Autodesk Inventor part; units mm, degrees
ref_plane "YZ Plane" through (0, 0, 0) normal (1, 0, 0) x (0, 1, 0)
ref_plane "XZ Plane" through (0, 0, 0) normal (0, 1, 0) x (-1, 0, 0)
ref_plane "XY Plane" through (0, 0, 0) normal (0, 0, 1) x (1, 0, 0)
sketch "스케치1" plane through (0, 0, 0) normal (0, 0, 1) x (1, 0, 0)
  line L0 (0, 0) -> (0, 150)
  line L1 (45, 0) -> (-45, 0)
  line L2 (-45, 0) -> (-45, 10)
  line L3 (-45, 10) -> (45, 10)
  line L4 (45, 10) -> (45, 0)
  line L5 (45, 0) -> (-45, 10) construction
  line L6 (-45, 0) -> (45, 10) construction
  line L7 (-35, 130) -> (35, 130)
  line L8 (35, 130) -> (35, 140)
  line L9 (35, 140) -> (-35, 140)
  line L10 (-35, 140) -> (-35, 130)
  line L11 (-35, 130) -> (35, 140) construction
  line L12 (35, 130) -> (-35, 140) construction
  line L13 (-40, 65) -> (40, 65)
  line L14 (40, 65) -> (40, 75)
  line L15 (40, 75) -> (-40, 75)
  line L16 (-40, 75) -> (-40, 65)
  line L17 (-40, 65) -> (40, 75) construction
  line L18 (40, 65) -> (-40, 75) construction
  line L19 (5, 150) -> (-5, 150)
  line L20 (-5, 0) -> (5, 0)
  line L21 (-45, 10) -> (-40, 10)
  line L22 (-40, 10) -> (-40, 75)
  line L23 (-40, 75) -> (-45, 75)
  line L24 (-45, 75) -> (-45, 10)
  line L25 (45, 10) -> (40, 10)
  line L26 (40, 10) -> (40, 75)
  line L27 (40, 75) -> (45, 75)
  line L28 (45, 75) -> (45, 10)
  line L29 (5, 0) -> (5, 10)
  line L30 (5, 65) -> (5, 150)
  line L31 (-5, 150) -> (-5, 65)
  line L32 (-5, 10) -> (-5, 0)
  line L33 (0, 10) -> (10, 10)
  line L34 (10, 10) -> (10, 65)
  line L35 (10, 65) -> (0, 65)
  line L36 (0, 65) -> (0, 10)
  line L37 (0, 10) -> (-10, 10)
  line L38 (-10, 10) -> (-10, 65)
  line L39 (-10, 65) -> (0, 65)
  line L40 (0, 65) -> (0, 10)
  line L41 (-10, 65) -> (-20, 65)
  line L42 (-20, 65) -> (-20, 10)
  line L43 (-20, 10) -> (-10, 10)
  line L44 (-10, 10) -> (-10, 65)
  line L45 (10, 65) -> (20, 65)
  line L46 (20, 65) -> (20, 10)
  line L47 (20, 10) -> (10, 10)
  line L48 (10, 10) -> (10, 65)
  point P0 (0, 5)
  point P1 (0, 135)
  point P2 (0, 70)
  point P3 (-5, 140)
  point P4 (5, 140)
  point P5 (-5, 75)
  point P6 (5, 75)
  point P7 (-5, 130)
  point P8 (5, 130)
  dimension "d16" = 150
  dimension "d17" = 90
  dimension "d18" = 10
  dimension "d22" = 70
  dimension "d23" = 10
  dimension "d25" = 80
  dimension "d26" = 10
  dimension "d27" = 55
  dimension "d28" = 55
  dimension "d29" = 10
  dimension "d30" = 150
  dimension "d35" = 10
  dimension "d36" = 10
  dimension "d37" = 10
  dimension "d38" = 10
extrude "돌출1" add sketch "스케치1" along normal blind 30 and the other way blind 30 contours L1 L32 L3 L0 | L0 L3 L29 L1 | L29 L3 L4 L1 | L1 L2 L3 L32 | L13 L31 L15 L0 | L0 L15 L30 L13 | L15 L31 L7 L0 | L0 L7 L30 L15 | L13 L16 L15 L31 | L30 L15 L14 L13 | L7 L31 L9 L0 | L0 L9 L30 L7 | L9 L31 L19 L0 | L0 L19 L30 L9 | L7 L10 L9 L31 | L30 L9 L8 L7
extrude "돌출2" add sketch "스케치1" along normal blind 30 and the other way blind 30 contours L3 L26 L14 L27 L28 | L24 L23 L16 L22 L3
extrude "돌출3" add sketch "스케치1" along normal blind 10 and the other way blind 10 contours L3 L42 L13 L38 | L34 L13 L46 L3
properties part number "팔"
Check sheet for the modelled part. Datum: model origin and axes. Units: mm. A direction names the side the tool comes from. Give positions to 0.01 mm unless a question says otherwise; leave off trailing zeros. Write each loop counter-clockwise with the first axis right and the second up, starting at its lowest first coordinate (ties: lowest second). Pieces come first, ordered by that corner, then holes.
Item 1: Scan lines: L1, parallel to Y at x = -24.5, z = -18; L2, parallel to X at y = 10.5, z = -4; L3, parallel to X at y = 30, z = -26.5. Record each from-to range of solid material in increasing order.
Item 2: Cross-section at B-B (z = -13). Enter the section's corners in (x, y), and give its area (3 significant figures).
Item 3: Cross-section at A-A (x = -23). Enter the section's corners in (y, z), and give its area (3 significant figures).
Item 4: Cross-section at D-D (x = -13.5). Enter the section's corners in (y, z).
Item 5: Access from +Z, -Z, +X, -X, +Y, -Y to the whole of each face (thin tool, end or side, straight path). Record for faces 4 (the face through (-20, 130, 0)), 5 (the face through (20, 140, 0)), 6 (the face through (15, 38, 10)).
Item 6: Draft check along Y on faces 1 (the face through (-20, 38, 0)), 2 (the face through (45, 38, 0)), 3 (the face through (-20, 140, 0)). Enter one of: released by +Y, released by -Y, zero draft, split by the parting line, or undercut.
Item 7: Gauge pin test, flat ends, axial feed: pin 1 (15 mm diameter, centred on x = 26, z = -7, fed in from +Y); pin 2 (1 mm diameter, centred on x = 19.5, y = 25, fed in from -Z); pin 3 (5 mm diameter, centred on y = 133.5, z = -0.5, fed in from +X). Record the tip position at first contact, or that the pin passes through.
Item 8: Cross-section at C-C (y = 20). Enter the section's corners in (x, z).
Report:
1. L1: y = 0 to 10, 65 to 75, 130 to 140
1. L2: x = -45 to -40, -20 to -10, 10 to 20, 40 to 45
1. L3: x = -45 to -40, 40 to 45
2. outline: (-45, 0) - (45, 0) - (45, 75) - (5, 75) - (5, 130) - (35, 130) - (35, 140) - (5, 140) - (5, 150) - (-5, 150) - (-5, 140) - (-35, 140) - (-35, 130) - (-5, 130) - (-5, 75) - (-45, 75) - close; hole (-40, 10) - (40, 10) - (40, 65) - (-40, 65) - close
2. area: 3,700 mm2
3. outline: (0, -30) - (10, -30) - (10, 30) - (0, 30) - close; (65, -30) - (75, -30) - (75, 30) - (65, 30) - close; (130, -30) - (140, -30) - (140, 30) - (130, 30) - close
3. area: 1,800 mm2
4. outline: (0, -30) - (10, -30) - (10, -10) - (65, -10) - (65, -30) - (75, -30) - (75, 30) - (65, 30) - (65, 10) - (10, 10) - (10, 30) - (0, 30) - close; (130, -30) - (140, -30) - (140, 30) - (130, 30) - close
5. face 4: +Z, -Z, -X
5. face 5: +Z, -Z, +X, +Y
5. face 6: +Z
6. face 1: undercut
6. face 2: zero draft
6. face 3: released by +Y
7. pin 1: stops at y = 140
7. pin 2: stops at z = -10
7. pin 3: stops at x = 35
8. outline: (-45, -30) - (-40, -30) - (-40, 30) - (-45, 30) - close; (-20, -10) - (-10, -10) - (-10, 10) - (-20, 10) - close; (10, -10) - (20, -10) - (20, 10) - (10, 10) - close; (40, -30) - (45, -30) - (45, 30) - (40, 30) - close
